Verification items for the finished model (mm, model axes). A direction names the side the tool comes from. Coordinates: 2 decimals unless noted, no trailing zeros. Write each loop counter-clockwise with the first axis right and the second up, starting at its lowest first coordinate (ties: lowest second). Pieces come first, ordered by that corner, then holes.
```python
from build123d import *

# Parameters (mm, degrees)
F0_R     = 2
F1_DEPTH = 2


with BuildPart() as f1:
    # F0 (on Front) → F1 (new body)
    with BuildSketch(Plane.XZ):
        with BuildLine():
            ThreePointArc((-0.487867, 5.820938), (-0.897138, 3.839724), (-2.05795, 2.182852))
            ThreePointArc((-2.05795, 2.182852), (0.018579, -2.999942), (2.030755, 2.208174))
            ThreePointArc((2.030755, 2.208174), (0.86277, 3.821091), (0.416949, 5.76195))
            Line((0.416949, 5.76195), (-0.487867, 41.509971))
            Line((-0.487867, 41.509971), (-0.487867, 5.820938))
        make_face()
        Circle(F0_R, mode=Mode.SUBTRACT)
    extrude(amount=F1_DEPTH)


solid = f1.part
```
1. Draft check along X on faces 3 (the cylindrical face through (0.874, -0.986, 3.796)), 4 (the flat face through (0, -2, 9)), 5 (the cylindrical face through (0, -1, -2)), 6 (the cylindrical face through (-0.886, -0.986, 3.866)). Enter one of: pulls with the +X half, pulls with the -X half, needs draft (parallel to the pull), parting line crosses it, or undercut.
2. Sectioned sample at D-D, the plane z = 8.5. Record the boundary of the cut face in (x, y).
3. Tool access check on faces 1 (the flat face through (-0.488, -1, 24)), 2 (the cylindrical face through (0, -1, -3)). Record the directions out of +Z, -Z, +X, -X, +Y, -Y that give a thin tool (end or side, any length) a straight path to the whole face; none if there is none.
4. Gauge pin test, flat end, axial feed: P1, Ø0.6, axis at y = -1, z = 24.5, coming from the -X side. Record the tip position at first contact, or that the pin passes through.
5. Sectioned sample at B-B, the plane x = -1.5. Record the boundary of the cut face in (y, z).
6. Sectioned sample at A-A, the plane z = 0. Record the boundary of the cut face in (x, y), and give its area (3 significant figures).
7. Material ranges on L1, parallel to Z at x = 1.65, y = -1.8; L2, parallel to Z at x = -1.6, y = -1.25; L3, parallel to X at y = -0.6, z = 22, recorded low to high.
8. Sectioned sample at C-C, the plane y = -1.65. Record the boundary of the cut face in (x, z), and give its area (3 significant figures).
Outcome:
1. face 3: pulls with the +X half
1. face 4: needs draft
1. face 5: undercut
1. face 6: pulls with the -X half
2. outline: (-0.49, -2) - (0.35, -2) - (0.35, 0) - (-0.49, 0) - close
3. face 1: +Z, -X, +Y, -Y
3. face 2: +Y, -Y
4. P1: stops at x = -0.49
5. outline: (-2, -2.6) - (0, -2.6) - (0, -1.32) - (-2, -1.32) - close; (-2, 1.32) - (0, 1.32) - (0, 2.8) - (-2, 2.8) - close
6. outline: (-3, -2) - (-2, -2) - (-2, 0) - (-3, 0) - close; (2, -2) - (3, -2) - (3, 0) - (2, 0) - close
6. area: 4.00 mm2
7. L1: z = -2.51 to -1.13, 1.13 to 2.6
7. L2: z = -2.54 to -1.2, 1.2 to 2.68
7. L3: x = -0.49 to 0.01
8. outline: (-2.06, 2.18) arc R3 ccw (long way) to (2.03, 2.21) arc R5 cw to (0.42, 5.76) - (-0.49, 41.51) - (-0.49, 5.82) arc R5 cw to start; hole circle Ø4 at (0, 0)
8. area: 36.4 mm2
